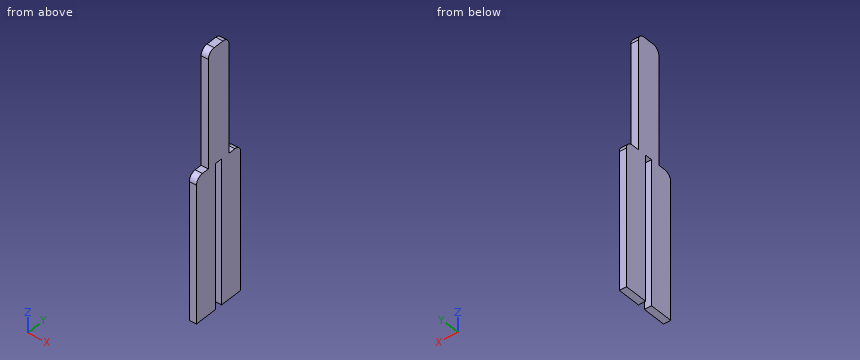
```python
from build123d import *

# Parameters (mm, degrees)
F1_DEPTH = 3.175


# Not quite as in the source:
# - ends of sketch curves that miss each other by under 0.0002 mm in the source are joined


with BuildPart() as f1:
    # F0 (on Right) → F1 (new body, symmetric)
    with BuildSketch(Plane.YZ):
        with BuildLine():
            Line((3.175, -63.5), (23.8125, -63.5))
            Line((23.8125, -63.5), (23.8125, 57.15))
            ThreePointArc((23.8125, 57.15), (21.9533763667, 61.6393796296), (17.4646167058, 63.4999996472))
            Line((17.4646167058, 63.4999996472), (17.4625, 63.5))
            Line((17.4625, 63.5), (11.1139111112, 63.5))
            Line((11.1139111112, 63.5), (11.124494366, 158.7492930333))
            ThreePointArc((11.124494366, 158.7492930333), (9.2648719104, 163.2398771909), (4.7744944052, 165.0999985889))
            Line((4.7744944052, 165.0999985889), (-4.7498, 165.0999985889))
            ThreePointArc((-4.7498, 165.0999985889), (-9.2399280605, 163.2401266494), (-11.0998, 158.7499985889))
            Line((-11.0998, 158.7499985889), (-11.0998, 63.5))
            Line((-11.0998, 63.5), (-17.4498, 63.5))
            Line((-17.4498, 63.5), (-17.4625, 63.5))
            ThreePointArc((-17.4625, 63.5), (-21.9526280605, 61.6401280605), (-23.8125, 57.15))
            Line((-23.8125, 57.15), (-23.8125, -63.5))
            Line((-23.8125, -63.5), (-3.175, -63.5))
            Line((-3.175, -63.5), (-3.175, 63.5))
            Line((-3.175, 63.5), (3.175, 63.5))
            Line((3.175, 63.5), (3.175, -63.5))
        make_face()
    extrude(amount=F1_DEPTH, both=True)


solid = f1.part
```
Source: CAD feature listing. Evaluate the final solid. Frame: model axes, mm. Give positions to 0.01 mm unless a question says otherwise; leave off trailing zeros. Loops run counter-clockwise (first coordinate to the right, second up) from the corner with the lowest first, then second, coordinate; pieces in that order, holes last. Notation, with made-up numbers: (-5.5, -22) -> (41.5, -22) arc R28 ccw to (41.5, 14) -> close; hole circle Ø3 at (29, 14). An arc over 180 degrees is marked (long way). Put each result on its own line as item: value. Start each with the question number.
1) Material intervals for probe 1 along Y at (x, z) = (1.25, -20.5) (1 decimal); probe 2 along Y at (x, z) = (-0.5, 108); probe 3 along Z at (x, y) = (-0.25, 12), sorted ascending.
2) Cut plane C-C (y = 0.5). Return loops of the section in (x, z) (3 decimals).
3) Cut plane A-A (z = 5.5). Return loops of the section in (x, y) (1 decimal).
4) Cut plane D-D (z = 61). Return loops of the section in (x, y) (3 decimals), then the cut area to 3 significant figures.
5) Contact query for flat-ended pins moving along their axis: P1, Ø2, axis at x = -2, y = 16.5, coming from the +Z side; P2, Ø3, axis at x = 0, z = 135, coming from the +Y side; P3, Ø1.9, axis at x = 1, y = -1, coming from the -Z side. Output: stop coordinate, or through.
Results are:
1. probe 1: y = -23.8 to -3.2, 3.2 to 23.8
1. probe 2: y = -11.1 to 11.12
1. probe 3: z = -63.5 to 63.5
2. outline: (-3.175, 63.5) -> (3.175, 63.5) -> (3.175, 165.1) -> (-3.175, 165.1) -> close
3. outline: (-3.2, -23.8) -> (3.2, -23.8) -> (3.2, -3.2) -> (-3.2, -3.2) -> close; (-3.2, 3.2) -> (3.2, 3.2) -> (3.2, 23.8) -> (-3.2, 23.8) -> close
4. outline: (-3.175, -22.512) -> (3.175, -22.512) -> (3.175, -3.175) -> (-3.175, -3.175) -> close; (-3.175, 3.175) -> (3.175, 3.175) -> (3.175, 22.512) -> (-3.175, 22.512) -> close
4. area: 246 mm2
5. P1: stops at z = 63.5
5. P2: stops at y = 11.12
5. P3: stops at z = 63.5
